```python
from build123d import *

# Parameters (mm, degrees)
ESQUISSE1_W                             = 13
ESQUISSE1_H                             = 55
BOSS_EXTRU_1_DEPTH                      = 8
TROUS_DE_CENTRAGE_5_0MMTRANSITIONAL_1_D = 5
ESQUISSE4_W                             = 4.5
ESQUISSE4_H                             = 20
ENL_V_MAT_EXTRU_1_DEPTH                 = 30.368350311
CONG_1_R                                = 2
CHANFREIN1_SIZE                         = 1
TROU_TARAUD_M41_D                       = 3.3
CHANFREIN2_START                        = -1
CHANFREIN2_DEPTH                        = 10
ESQUISSE9_W                             = 8
ESQUISSE9_H                             = 8
ENL_V_MAT_EXTRU_2_DEPTH                 = 30.874738493
ESQUISSE10_W                            = 4
ESQUISSE10_H                            = 8
BOSS_EXTRU_2_DEPTH                      = 7
CHANFREIN3_SIZE                         = 1
BOSS_EXTRU_3_START                      = -8
BOSS_EXTRU_3_DEPTH                      = 8
CONG_2_R                                = 8


with BuildPart() as part:
    # Esquisse1 → Boss.-Extru.1 (new body)
    with BuildSketch(Plane.XY):
        Rectangle(ESQUISSE1_W, ESQUISSE1_H)
    extrude(amount=BOSS_EXTRU_1_DEPTH)

    # Trous de centrage Ø5.0mmTransitional 1 (through all)
    with Locations(Plane.XY.offset(8)):
        with Locations((0, 0.5)):
            Hole(TROUS_DE_CENTRAGE_5_0MMTRANSITIONAL_1_D / 2)

    # Esquisse4 → Enlèv. mat.-Extru.1 (cut, through all)
    with BuildSketch(Plane.XY.offset(8)):
        with Locations((4.25, 17.5)):
            Rectangle(ESQUISSE4_W, ESQUISSE4_H)
        with Locations((-4.25, 17.5)):
            Rectangle(ESQUISSE4_W, ESQUISSE4_H)
    extrude(amount=-ENL_V_MAT_EXTRU_1_DEPTH, mode=Mode.SUBTRACT)

    # Congé1
    cong_1_edges = [part.edges().sort_by_distance(p)[0] for p in [
        (2, 7.5, 4),
        (-2, 7.5, 4),
    ]]
    fillet(cong_1_edges, radius=CONG_1_R)

    # Chanfrein1
    chanfrein1_edges = [part.edges().sort_by_distance(p)[0] for p in [
        (6.5, -27.5, 4),
        (-6.5, -27.5, 4),
    ]]
    chamfer(chanfrein1_edges, length=CHANFREIN1_SIZE)

    # Trou taraudé M41 (through all)
    with Locations(Plane.XY.offset(8)):
        with Locations((-3.775, -23.5), (3.775, -23.5)):
            Hole(TROU_TARAUD_M41_D / 2)

    # Chanfrein2: read off the stored shape, not the designer's step
    # Chanfrein2 outline → Chanfrein2 (cut)
    with BuildSketch(Plane.XY.offset(CHANFREIN2_START)):
        with BuildLine():
            Line((3.285714286, 7.631900453), (6.5, 2.961651585))
            Line((6.5, 2.961651585), (6.5, 7.5))
            Line((6.5, 7.5), (4, 7.5))
            ThreePointArc((4, 7.5), (3.636818981, 7.533251529), (3.285714286, 7.631900453))
        make_face()
        with BuildLine():
            Line((-6.5, 2.961651585), (-3.285714286, 7.631900453))
            ThreePointArc((-3.285714286, 7.631900453), (-3.636818981, 7.533251529), (-4, 7.5))
            Line((-4, 7.5), (-6.5, 7.5))
            Line((-6.5, 7.5), (-6.5, 2.961651585))
        make_face()
    extrude(amount=CHANFREIN2_DEPTH, mode=Mode.SUBTRACT)

    # Esquisse9 → Enlèv. mat.-Extru.2 (cut, through all)
    with BuildSketch(Plane.ZY.offset(2)):
        with Locations((4, 23.5)):
            Rectangle(ESQUISSE9_W, ESQUISSE9_H)
    extrude(amount=-ENL_V_MAT_EXTRU_2_DEPTH, mode=Mode.SUBTRACT)

    # Esquisse10 → Boss.-Extru.2 (add)
    with BuildSketch(Plane(origin=(0, 19.5, 0), x_dir=(1, 0, 0), z_dir=(0, 1, 0))):
        with Locations((0, -4)):
            Rectangle(ESQUISSE10_W, ESQUISSE10_H)
    extrude(amount=BOSS_EXTRU_2_DEPTH)

    # Chanfrein3
    chanfrein3_edges = [part.edges().sort_by_distance(p)[0] for p in [
        (0, 26.5, 0),
        (0, 26.5, 8),
    ]]
    chamfer(chanfrein3_edges, length=CHANFREIN3_SIZE)

    # Esquisse11 → Boss.-Extru.3 (add)
    with BuildSketch(Plane.XY.offset(8).offset(BOSS_EXTRU_3_START)):
        with BuildLine():
            Line((-3.285714286, 7.631900453), (-2, 9.5))
            ThreePointArc((-2, 9.5), (-2.352491058, 8.366106581), (-3.285714286, 7.631900453))
        make_face()
        with BuildLine():
            Line((3.285714286, 7.631900453), (2, 9.5))
            ThreePointArc((2, 9.5), (2.352491058, 8.366106581), (3.285714286, 7.631900453))
        make_face()
    extrude(amount=BOSS_EXTRU_3_DEPTH)

    # Congé2
    cong_2_edges = [part.edges().sort_by_distance(p)[0] for p in [
        (-2, 9.5, 4),
        (2, 9.5, 4),
    ]]
    fillet(cong_2_edges, radius=CONG_2_R)


solid = part.part
```
Build history of the part. All positions in model axes, mm. A direction names the side the tool comes from. Round coordinates to 2 decimals unless told otherwise and drop trailing zeros. Write each loop counter-clockwise with the first axis right and the second up, starting at its lowest first coordinate (ties: lowest second). Pieces come first, ordered by that corner, then holes.
1) Drill centre lines: probe 1 along Y at (x, z) = (0, 4.75); probe 2 along Y at (x, z) = (4.5, 5.5); probe 3 along X at (y, z) = (14, 3). Where is each one in solid material? Low to high.
2) Band-saw the part on D-D, the plane z = 4.25. Give the number of separate pieces and of enclosed holes in the cut face, and give its area (3 significant figures).
3) Band-saw the part on B-B, the plane y = 0.5. List the corners of the cut face in (x, z).
4) Mould opens along X. For faces 1 (the cylindrical face through (-1.34, 2.61, 3.94)), 2 (the flat face through (-4.977, 5.175, 3.944)), 3 (the flat face through (0, 26, 7.5)) say: +X half, -X half, draft (parallel to the pull), parting line (faces both ways), or undercut.
5) 3-axis set-ups, long thin cutter, end or side, ignore diameter. For faces 4 (the flat face through (-6.5, -12, 4)), 5 (the flat face through (-2, 19, 4)), 6 (the flat face through (2, 19, 4)): which of +Z, -Z, +X, -X, +Y, -Y reach the whole face in a straight line?
6) Band-saw the part on A-A, the plane x = 0. List the corners of the cut face in (y, z), and give its area (3 significant figures).
7) Band-saw the part on C-C, the plane y = -23.5. List the corners of the cut face in (x, z) (3 decimals).
Ans:
1. probe 1: y = -27.5 to -2, 3 to 26.5
1. probe 2: y = -27.5 to -24.98, -22.02 to 5.87
1. probe 3: x = -2 to 2
2. separate pieces: 1
2. enclosed holes: 3
2. area: 483 mm2
3. outline: (-6.5, 0) - (-2.5, 0) - (-2.5, 8) - (-6.5, 8) - close; (2.5, 0) - (6.5, 0) - (6.5, 8) - (2.5, 8) - close
4. face 1: undercut
4. face 2: -X half
4. face 3: draft
5. face 4: +Z, -Z, -X, +Y, -Y
5. face 5: +Z, -Z, -X, +Y
5. face 6: +Z, -Z, +X, +Y
6. outline: (-27.5, 0) - (-2, 0) - (-2, 8) - (-27.5, 8) - close; (3, 0) - (25.5, 0) - (26.5, 1) - (26.5, 7) - (25.5, 8) - (3, 8) - close
6. area: 391 mm2
7. outline: (-6.5, 0) - (-5.425, 0) - (-5.425, 8) - (-6.5, 8) - close; (-2.125, 0) - (2.125, 0) - (2.125, 8) - (-2.125, 8) - close; (5.425, 0) - (6.5, 0) - (6.5, 8) - (5.425, 8) - close
